The model under review builds one solid part; all positions refer to its coordinate system, in mm. A direction names the side the tool comes from. Give positions to 0.01 mm unless a question says otherwise; leave off trailing zeros. Order: outer loops, then holes, each group sorted by start corner. A loop starts at its lowest first (then second) coordinate and runs counter-clockwise, first axis right, second up. Notation, with made-up numbers: (57, -26) - (74, -26) arc R18 cw to (74, -21) - close; hole circle Ø2 at (-20, -31). An arc over 180 degrees is marked (long way). Use a Markdown table: item, result. Add a question column.
```python
from build123d import *

# Parameters (mm, degrees)
F0_R     = 3.4036
F1_DEPTH = 31.75
F2_R     = 2.0066
F3_DEPTH = 23.114
F7_R     = 0.381
F8_SIZE  = 0.254


with BuildPart() as f1:
    # F0 (on Top) → F1 (new body)
    with BuildSketch(Plane.XY):
        Circle(F0_R)
    extrude(amount=F1_DEPTH)

    # F2 (on face) → F3 (cut)
    with BuildSketch(Plane.XY.offset(31.75)):
        Circle(F2_R)
    extrude(amount=-F3_DEPTH, mode=Mode.SUBTRACT)

    # F5 (on offset) → F6 (revolve, cut)
    with BuildSketch(Plane(origin=(0, 0, -0.508), x_dir=(1, 0, 0), z_dir=(0, 0, -1))):
        with BuildLine():
            ThreePointArc((0, 1.651), (-1.651, 0), (0, -1.651))
            Line((0, -1.651), (0, 1.651))
        make_face()
    revolve(axis=Axis((0, -0.148408, -0.508), (0, -1, 0)), mode=Mode.SUBTRACT)

    # F7
    f7_edges = [f1.edges().sort_by_distance(p)[0] for p in [
        (-3.4036, 0, 0),
    ]]
    fillet(f7_edges, radius=F7_R)

    # F8
    f8_edges = [f1.edges().sort_by_distance(p)[0] for p in [
        (-3.4036, 0, 31.75),
        (-2.0066, 0, 31.75),
    ]]
    chamfer(f8_edges, length=F8_SIZE)


solid = f1.part
```
Q1. Machinability: for faces 4 (the cylindrical face through (-1.479, 1.356, 20.226)), 5 (the flat face through (1.3, -1.3, 0)), which of the approach directions +Z, -Z, +X, -X, +Y, -Y give a long, thin tool a straight path to every point of the face, cutting with its end or side? Answer none if there is none.
Q2. Draft analysis for pull direction X (two halves, no side actions). For faces 1 (the cylindrical face through (3.144, -1.304, 15.721)), 2 (the flat face through (1.4, -2.1, 31.75)), 3 (the flat face through (0, 0, 8.636)), state which applies: pulls with the +X half, pulls with the -X half, needs draft (parallel to the pull), parting line crosses it, or undercut.
Q3. Wall thickness on probe 1 along Y at (x, z) = (0, 20); probe 2 along Z at (x, y) = (-1.25, 1.5); probe 3 along Y at (x, z) = (-1.5, 23): over which ranges is each line inside the solid? List them lowest first.
Q4. We need section C-C (z = 29). Write out the cut boundary in (x, y), plus the area to 3 significant figures.
Q5. We need section D-D (z = 6). Write out the cut boundary in (x, y), plus the area to 3 significant figures.
Q6. We need section A-A (x = 0). Write out the cut boundary in (y, z), plus the area to 3 significant figures.
Q7. Clearance check with flat-ended pins moving along their axes: P1, Ø3, axis at x = -2.5, z = 6, coming from the +Y side; P2, Ø3.5, axis at x = 0, y = 0, coming from the +Z side. State where each tip first meets the part, or that it passes through.
Here are the results:
| question | item | result |
|---|---|---|
| 1 | face 4 | +Z |
| 1 | face 5 | -Z, +X, -X, +Y, -Y |
| 2 | face 1 | parting line crosses it |
| 2 | face 2 | needs draft |
| 2 | face 3 | undercut |
| 3 | probe 1 | -3.4 to -2.01, 2.01 to 3.4 |
| 3 | probe 2 | 0 to 8.64 |
| 3 | probe 3 | -3.06 to -1.33, 1.33 to 3.06 |
| 4 | outline | circle Ø6.81 at (0, 0); hole circle Ø4.01 at (0, 0) |
| 4 | area | 23.7 mm2 |
| 5 | outline | circle Ø6.81 at (0, 0) |
| 5 | area | 36.4 mm2 |
| 6 | outline | (-3.4, 0.38) arc R0.38 ccw to (-3.02, 0) - (-1.57, 0) arc R1.65 cw to (1.57, 0) - (3.02, 0) arc R0.38 ccw to (3.4, 0.38) - (3.4, 31.5) - (3.15, 31.75) - (2.26, 31.75) - (2.01, 31.5) - (2.01, 8.64) - (-2.01, 8.64) - (-2.01, 31.5) - (-2.26, 31.75) - (-3.15, 31.75) - (-3.4, 31.5) - close |
| 6 | area | 121 mm2 |
| 7 | P1 | y = 3.25 |
| 7 | P2 | z = 8.64 |
